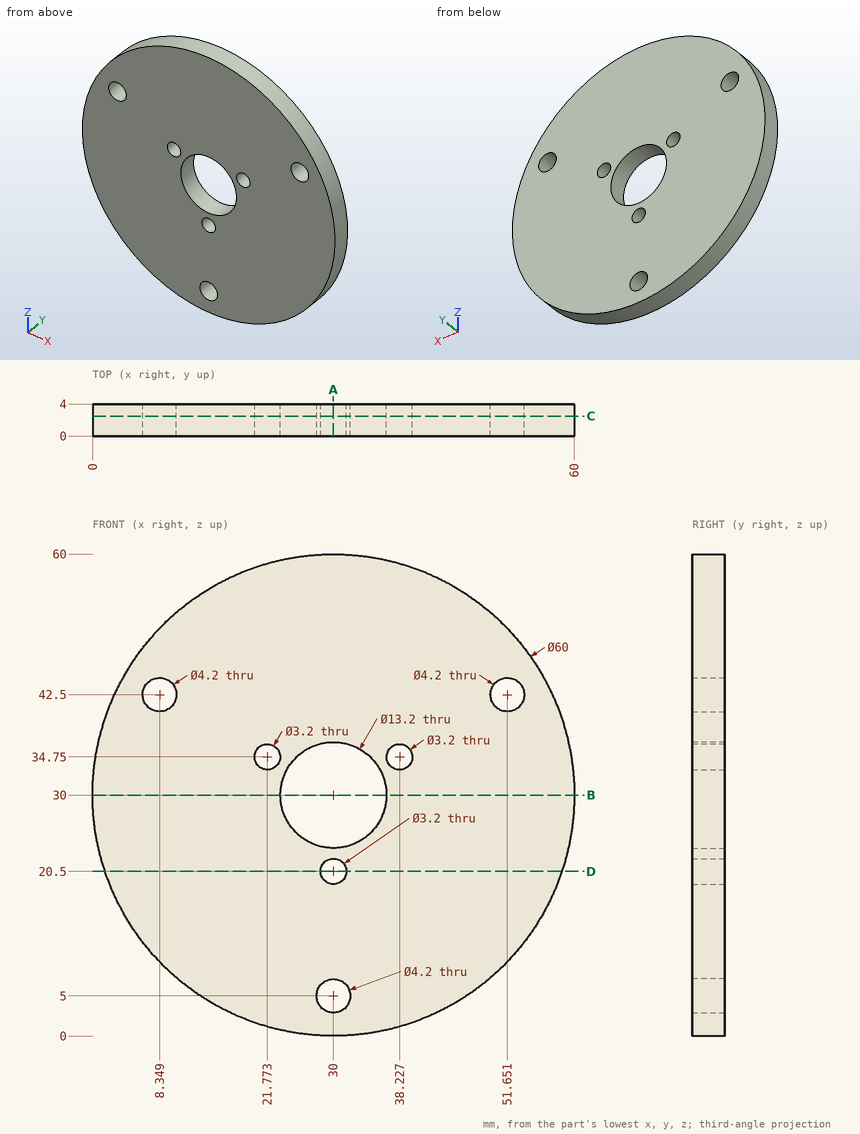
Source: three-view drawing plus pictorial views. Frame: mm from the lowest corner of the part. Give positions to 0.01 mm unless a question says otherwise; leave off trailing zeros. Loops run counter-clockwise (first coordinate to the right, second up) from the corner with the lowest first, then second, coordinate; pieces in that order, holes last.
1) Section query A-A on x = 30. Return the cut outline in (y, z).
A:
outline: (0, 0) - (4, 0) - (4, 2.9) - (0, 2.9) - close; (0, 7.1) - (4, 7.1) - (4, 18.9) - (0, 18.9) - close; (0, 22.1) - (4, 22.1) - (4, 23.4) - (0, 23.4) - close; (0, 36.6) - (4, 36.6) - (4, 60) - (0, 60) - close
2) Section query C-C on y = 2.5. Count the separate pieces of the cut face and the enclosed holes in it, and give its area (4 significant figures).
A:
separate pieces: 1
enclosed holes: 7
area: 2,625 mm2
3) Line query: L1, parallel to X at y = 1.45, z = 30; L2, parallel to X at y = 1.75, z = 42.5; L3, parallel to X at y = 1.55, z = 34.75 (1 decimal). Output: solid intervals per line, ascending.
A:
L1: x = 0 to 23.4, 36.6 to 60
L2: x = 2.73 to 6.25, 10.45 to 49.55, 53.75 to 57.27
L3: x = 0.4 to 20.2, 23.4 to 25.4, 34.6 to 36.6, 39.8 to 59.6
4) Contact query for flat-ended pins moving along their axis: pin 1 (2 mm diameter, centred on x = 37, y = 3.5, fed in from -Z); pin 2 (2 mm diameter, centred on x = 44, y = 2, fed in from +Z). Output: stop coordinate, or through.
A:
pin 1: stops at z = 0.61
pin 2: stops at z = 57.04
5) Section query D-D on z = 20.5. Return the cut outline in (x, y), and give its area (3 significant figures).
A:
outline: (1.54, 0) - (28.4, 0) - (28.4, 4) - (1.54, 4) - close; (31.6, 0) - (58.46, 0) - (58.46, 4) - (31.6, 4) - close
area: 215 mm2
6) Section query B-B on z = 30. Return the cut outline in (x, y).
A:
outline: (0, 0) - (23.4, 0) - (23.4, 4) - (0, 4) - close; (36.6, 0) - (60, 0) - (60, 4) - (36.6, 4) - close
